Read the model definition and answer for the solid it produces. Units are mm, in the model's axes. A direction names the side the tool comes from. Coordinates: 2 decimals unless noted, no trailing zeros. Loops run counter-clockwise (first coordinate to the right, second up) from the corner with the lowest first, then second, coordinate; pieces in that order, holes last. Notation, with made-up numbers: (13.25, 20.25) - (41.25, 20.25) arc R15 cw to (41.25, 34.25) - close; hole circle Ø2 at (57.25, -8). An arc over 180 degrees is marked (long way). Use CSV: the item, a comma, the result in double quotes.
Autodesk Inventor part; units mm, degrees
ref_plane "YZ Plane" through (0, 0, 0) normal (1, 0, 0) x (0, 1, 0)
ref_plane "XZ Plane" through (0, 0, 0) normal (0, 1, 0) x (-1, 0, 0)
ref_plane "XY Plane" through (0, 0, 0) normal (0, 0, 1) x (1, 0, 0)
sketch "Sketch1" plane through (0, 0, 0) normal (0, 1, 0) x (-1, 0, 0)
  circle A0 centre (0, 0) radius 60
  dimension "d0" = 120
extrude "Extrusion1" add sketch "Sketch1" along normal blind 15
sketch "Sketch2" plane through (0, 15, 0) normal (0, 1, 0) x (1, 0, 0)
  circle A0 centre (0, 0) radius 52.5
  circle A1 centre (0, 0) radius 47.5
  dimension "d3" = 105
  dimension "d4" = 95
extrude "Extrusion2" cut sketch "Sketch2" against normal blind 10
sketch "Sketch3" plane through (0, 15, 0) normal (0, 1, 0) x (1, 0, 0)
  circle A0 centre (0, 0) radius 55
  circle A1 centre (0, 0) radius 54
  dimension "d7" = 110
  dimension "d8" = 108
extrude "Extrusion3" cut sketch "Sketch3" against normal blind 10
properties part number "pathBase" material "Stainless Steel"
Q1. A tool of negligible diameter and unlimited length cuts with its end or side. For faces 5 (the face through (8.3, 15, 52.3)), 6 (the face through (-11.9, 5, 46.4)), from which of +Z, -Z, +X, -X, +Y, -Y can it reach the whole face along a straight path? Write none if from no direction.
Reported:
face 5,"+Z, -Z, +X, -X, +Y"
face 6,"+Y"
Q2. Given P1, Ø2, axis at x = 5, y = 5.5, coming from the -Z side; P2, Ø5, axis at x = -12.5, y = 12.5, coming from the -Z side; P3, Ø3, axis at x = -14.5, y = 8.5, coming from the +Z side, each flat-ended and moving along its own axis, determine where each tip first touches the part or whether it passes through.
Reported:
P1,"stops at z = -59.87"
P2,"stops at z = -59.16"
P3,"stops at z = 58.57"
Q3. Find the intervals of material crossed by probe 1 along Z at (x, y) = (0, 7.75); probe 2 along Z at (x, y) = (-31.5, 12.25); probe 3 along X at (y, z) = (10.75, -16), in increasing order. Write a range as [from, to].
Reported:
probe 1,"z = [-60, -55], [-54, -52.5], [-47.5, 47.5], [52.5, 54], [55, 60]"
probe 2,"z = [-51.07, -45.09], [-43.86, -42], [-35.55, 35.55], [42, 43.86], [45.09, 51.07]"
probe 3,"x = [-57.83, -52.62], [-51.58, -50], [-44.72, 44.72], [50, 51.58], [52.62, 57.83]"
Q4. The part is cut by section C-C on z = 0. Determine the outline of the cut face in (x, y), and give its area (3 significant figures).
Reported:
outline,"(-60, 0) - (60, 0) - (60, 15) - (55, 15) - (55, 5) - (54, 5) - (54, 15) - (52.5, 15) - (52.5, 5) - (47.5, 5) - (47.5, 15) - (-47.5, 15) - (-47.5, 5) - (-52.5, 5) - (-52.5, 15) - (-54, 15) - (-54, 5) - (-55, 5) - (-55, 15) - (-60, 15) - close"
area,"1,680 mm²"
Q5. The part is cut by section B-B on x = 0. Determine the outline of the cut face in (y, z).
Reported:
outline,"(0, -60) - (15, -60) - (15, -55) - (5, -55) - (5, -54) - (15, -54) - (15, -52.5) - (5, -52.5) - (5, -47.5) - (15, -47.5) - (15, 47.5) - (5, 47.5) - (5, 52.5) - (15, 52.5) - (15, 54) - (5, 54) - (5, 55) - (15, 55) - (15, 60) - (0, 60) - close"
Q6. For a pull along X with two mould halves and no side action, classify faces 1 (the face through (-11.923, 10.07, 53.692)), 2 (the face through (-26, 15, -49)), 3 (the face through (-10.3, 10.07, 46.37)), 4 (the face through (59.94, 7.4, -2.64)) as +X half, -X half, draft (parallel to the pull), parting line (faces both ways), or undercut.
Reported:
face 1,"undercut"
face 2,"draft"
face 3,"undercut"
face 4,"parting line"
Q7. The part is cut by section A-A on y = 7.75. Determine the outline of the cut face in (x, z).
Reported:
outline,"circle Ø120 at (0, 0); circle Ø108 at (0, 0); circle Ø95 at (0, 0); hole circle Ø110 at (0, 0); hole circle Ø105 at (0, 0)"
